Autodesk Inventor part; units mm, degrees
ref_plane "YZ Plane" through (0, 0, 0) normal (1, 0, 0) x (0, 1, 0)
ref_plane "XZ Plane" through (0, 0, 0) normal (0, 1, 0) x (-1, 0, 0)
ref_plane "XY Plane" through (0, 0, 0) normal (0, 0, 1) x (1, 0, 0)
ref_plane "Work Plane1" through (0, 0, -28) normal (0, 0, 1) x (1, 0, 0)
sketch "Sketch1" plane through (0, 0, -28) normal (0, 0, 1) x (1, 0, 0)
  circle A0 centre (27.88, 8) radius 2.6486
  circle A1 centre (27.88, 43) radius 2.6486
  circle A2 centre (44.7, 24.3248) radius 2.6486
  line L0 (27.88, 8) -> (44.7, 24.3248)
  line L1 (44.7, 24.3248) -> (27.88, 43)
  line L2 (27.88, 43) -> (27.88, 8)
  line L3 (46.5446, 22.4242) -> (29.7246, 6.0994)
  line L4 (46.668, 26.0973) -> (29.848, 44.7725)
  line L5 (27.88, 5.3514) -> (11.88, 5.3514)
  line L6 (27.88, 5.3514) -> (43.88, 5.3514) construction
  line L7 (11.88, 5.3514) -> (11.88, 45.6486)
  line L8 (11.88, 45.6486) -> (27.88, 45.6486)
  point P0 (0, 0)
  dimension "d0" = 16
  dimension "d1" = 180
extrude "Extrusion1" add sketch "Sketch1" along normal blind 1
sketch "Sketch2" plane through (0, 0, -28) normal (0, 0, -1) x (-1, 0, 0)
  circle A0 centre (-44.7, 24.3248) radius 2.6486
  circle A1 centre (-27.88, 43) radius 2.6486
  circle A2 centre (-27.88, 8) radius 2.6486
  point P0 (0, 0)
extrude "Extrusion2" add sketch "Sketch2" along normal blind 2 draft -40
properties part number "20_Cube_Insert_VCM_MirrorMount_KES400A_mirror_mount"
The listing builds one solid part. Answer for the finished solid, in the listing's coordinates (mm). Give positions to 0.01 mm unless a question says otherwise; leave off trailing zeros. Write each loop counter-clockwise with the first axis right and the second up, starting at its lowest first coordinate (ties: lowest second). Pieces come first, ordered by that corner, then holes. Notation, with made-up numbers: (-10.75, 7) -> (6.25, 7) arc R6 ccw to (6.25, 13) -> close; hole circle Ø8 at (-23, 88). An arc over 180 degrees is marked (long way). Write item = value, one per line. Start each with the question number.
1) Straight lines are drawn through the part: line 1 along Z through (x, y) = (23, 18.5); line 2 along X through (y, z) = (42, -29.45); line 3 along X through (y, z) = (25.5, -28.15). For each, find the intervals that lie inside material, in ascending order.
2) The part is cut by section D-D, the plane x = 14.5. Determine the outline of the cut face in (y, z), and give its area (3 significant figures).
3) The part is cut by section A-A, the plane x = 44.7. Determine the outline of the cut face in (y, z).
4) Determine the mould class of faces 1 (the face through (19.8, 45.649, -27.5)), 2 (the face through (26.85, 7.68, -29.87)), 3 (the face through (26.887, 43.412, -29.875)), 4 (the face through (47.348, 24.264, -27.507)) for opening direction Y: +Y half, -Y half, draft (parallel to the pull), parting line (faces both ways), or undercut.
5) The part is cut by section B-B, the plane y = 8. Determine the outline of the cut face in (x, z), and give its area (3 significant figures).
6) The part is cut by section C-C, the plane z = -28.9. Determine the outline of the cut face in (x, y), and give its area (3 significant figures).
7) This flat-tipped pin is pushed along its axis until it touches: pin 1 (1 mm diameter, centred on x = 33.5, y = 14.5, fed in from -Z). Where does it stop, or does it pass through?
Solutions:
q1.line_1 = -28 to -27
q1.line_2 = 26.86 to 28.9
q1.line_3 = 42.47 to 46.93
q2.outline = (5.35, -28) -> (45.65, -28) -> (45.65, -27) -> (5.35, -27) -> close
q2.area = 40.3 mm²
q3.outline = (20.63, -28) -> (21.68, -28) -> (23.35, -30) -> (25.3, -30) -> (26.97, -28) -> (28.28, -28) -> (28.28, -27) -> (20.63, -27) -> close
q4.face_1 = +Y half
q4.face_2 = undercut
q4.face_3 = undercut
q4.face_4 = parting line
q5.outline = (11.88, -28) -> (25.23, -28) -> (26.91, -30) -> (28.85, -30) -> (30.53, -28) -> (31.68, -28) -> (31.68, -27) -> (11.88, -27) -> close
q5.area = 27.0 mm²
q6.outline = circle Ø3.79 at (27.88, 8); circle Ø3.79 at (27.88, 43); circle Ø3.79 at (44.7, 24.32)
q6.area = 33.8 mm²
q7.pin_1 = -28
